Input: part model. Units: mm. Frame: model coordinates. Face numbers are marked on the shaded views. Coordinates: 2 decimals unless noted, no trailing zeros. Loops run counter-clockwise (first coordinate to the right, second up) from the corner with the lowest first, then second, coordinate; pieces in that order, holes last. Notation, with made-up numbers: M 67.5,70.5 L 119.5,70.5 A29 cw 119.5,105.5 Z; hole C 83,-9 d9. An arc over 180 degrees is marked long. Use a Markdown table: item, result. Add a question column.
1. Draft query along Z for the marked faces 1, 2 and 3. Return one class per face: +Z half, -Z half, draft (parallel to the pull), parting line (faces both ways), or undercut.
2. Section C-C on x = -177. Output: boundary loops of the cut face in (y, z), then the cut area to 3 significant figures.
3. Section A-A on x = -367. Output: boundary loops of the cut face in (y, z).
4. Line query: L1, parallel to X at y = -75.5, z = -18; L2, parallel to X at y = -59, z = -19; L3, parallel to Y at x = -282, z = -8. Output: solid intervals per line, ascending. Write a range as [from, to].
5. Section B-B on y = -24.5. Output: boundary loops of the cut face in (x, z).
6. Pin query (flat end, axial travel): pin 1 (12 mm diameter, centred on y = -91, z = -15.5, fed in from -X); pin 2 (2 mm diameter, centred on y = -32.5, z = -8.5, fed in from -X); pin 3 (10 mm diameter, centred on x = -361.5, z = -10.5, fed in from +Y). Return the tip coordinate at first contact, or that it passes through.
```python
from build123d import *

# Parameters (mm, degrees)
SKETCH1_W           = 325
SKETCH1_H           = 60
BOSS_EXTRUDE1_DEPTH = 114.37
SKETCH2_R           = 17.238668945
BOSS_EXTRUDE2_DEPTH = 25
SKETCH3_R           = 1
BOSS_EXTRUDE3_DEPTH = 355.6


with BuildPart() as part:
    # Sketch1 → Boss-Extrude1 (new body)
    with BuildSketch(Plane(origin=(0, 0, 0), x_dir=(1, 0, 0), z_dir=(0, 1, 0))):
        Rectangle(SKETCH1_W, SKETCH1_H)
    extrude(amount=-BOSS_EXTRUDE1_DEPTH)

    # Sketch2 → Boss-Extrude2 (add)
    with BuildSketch(Plane.ZY.offset(162.5)):
        with Locations((-7.5, -49.37)):
            Circle(SKETCH2_R)
    extrude(amount=BOSS_EXTRUDE2_DEPTH)

    # Sketch3 → Boss-Extrude3 (add)
    with BuildSketch(Plane.ZY.offset(187.5)):
        with Locations((-7.5, -49.37)):
            Circle(SKETCH3_R)
    extrude(amount=BOSS_EXTRUDE3_DEPTH)


solid = part.part
```
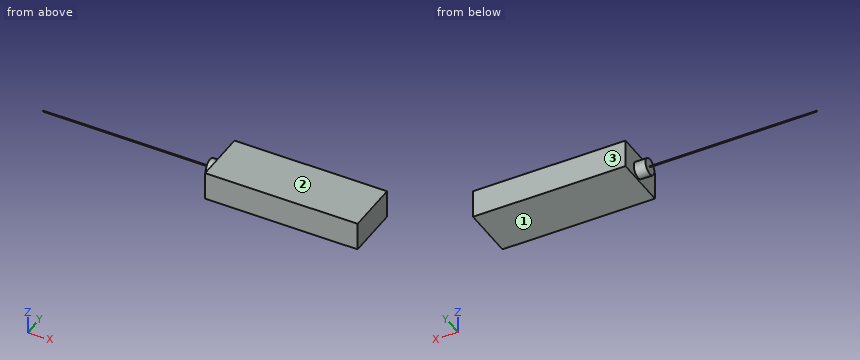
Answers below:
| question | item | result |
|---|---|---|
| 1 | face 1 | -Z half |
| 1 | face 2 | +Z half |
| 1 | face 3 | draft |
| 2 | outline | C -49.37,-7.5 d34.48 |
| 2 | area | 934 mm² |
| 3 | outline | C -49.37,-7.5 d2 |
| 4 | L1 | x = [-162.5, 162.5] |
| 4 | L2 | x = [-187.5, 162.5] |
| 4 | L3 | y = [-50.24, -48.5] |
| 5 | outline | M -162.5,-30 L 162.5,-30 L 162.5,30 L -162.5,30 Z |
| 6 | pin 1 | stops at x = -162.5 |
| 6 | pin 2 | stops at x = -187.5 |
| 6 | pin 3 | stops at y = -48.37 |
